Verification items for the finished model (mm, model axes). A direction names the side the tool comes from. Round coordinates to 2 decimals unless told otherwise and drop trailing zeros. Order: outer loops, then holes, each group sorted by start corner. A loop starts at its lowest first (then second) coordinate and runs counter-clockwise, first axis right, second up. Notation, with made-up numbers: M -23.5,53.5 L 32.5,53.5 A15 cw 32.5,62.5 Z; hole C -5,1.5 d11. An arc over 180 degrees is marked long. One line per item, written item: value. Start each with the question number.
from build123d import *

# Parameters (mm, degrees)
F0_R     = 9
F1_DEPTH = 15.3
F2_SIZE  = 1
F3_SIZE2 = 1.5
F3_SIZE  = 1
F4_R     = 3.5
F5_DEPTH = 2
F6_R     = 2.4
F7_DEPTH = 12.5
F8_R     = 1
F9_DEPTH = 1.5


with BuildPart() as f1:
    # F0 (on Top) → F1 (new body)
    with BuildSketch(Plane.XY):
        Circle(F0_R)
    extrude(amount=F1_DEPTH)

    # F2
    f2_edges = [f1.edges().sort_by_distance(p)[0] for p in [
        (-9, 0, 0),
    ]]
    chamfer(f2_edges, length=F2_SIZE)

    # F3
    f3_edges = [f1.edges().sort_by_distance(p)[0] for p in [
        (-9, 0, 15.3),
    ]]
    f3_side = f1.faces().sort_by_distance((0, 0, 15.3))[0]
    chamfer(f3_edges, length=F3_SIZE, length2=F3_SIZE2, reference=f3_side)

    # F4 (on face) → F5 (join)
    with BuildSketch(Plane.XY.offset(15.3)):
        Circle(F4_R)
    extrude(amount=F5_DEPTH)

    # F6 (on face) → F7 (join)
    with BuildSketch(Plane.XY.offset(17.3)):
        Circle(F6_R)
    extrude(amount=F7_DEPTH)

    # F8 (on face) → F9 (join)
    with BuildSketch(Plane(origin=(0, 0, 0), x_dir=(1, 0, 0), z_dir=(0, 0, -1))):
        Circle(F8_R)
    extrude(amount=F9_DEPTH)


solid = f1.part
1. Section check D-D (z = 21.5). Record the cut outline in (x, y), and give its area (3 significant figures).
2. Section check A-A (y = 0). Record the cut outline in (x, z).
3. Depth check by flat-ended pin: pin 1 (6 mm diameter, centred on y = -5.5, z = 21, fed in from +X); pin 2 (4 mm diameter, centred on x = -5, y = -7, fed in from +Z); pin 3 (5 mm diameter, centred on x = 6, y = -2.5, fed in from -Z); pin 4 (1.5 mm diameter, centred on y = 4, z = 15, fed in from +X). Enter the tip coordinate at first touch or a pass-through.
4. Tool access check on faces 1 (the face through (0, 1, -1)), 2 (the face through (1.29, 2.024, 23.462)), 3 (the face through (-1.172, 8.923, 7.31)). Record the directions out of +Z, -Z, +X, -X, +Y, -Y that give a thin tool (end or side, any length) a straight path to the whole face; none if there is none.
5. Scan lines: line 1 along Z through (x, y) = (-7.5, 0.25); line 2 along Z through (x, y) = (-1, 1.75); line 3 along Y through (x, z) = (-3.25, 2). Record each from-to range of solid material in increasing order.
6. Section check C-C (z = 2). Record the cut outline in (x, y), and give its area (3 significant figures).
Geometry check:
1. outline: C 0,0 d4.8
1. area: 18.1 mm²
2. outline: M -9,1 L -8,0 L -1,0 L -1,-1.5 L 1,-1.5 L 1,0 L 8,0 L 9,1 L 9,13.8 L 8,15.3 L 3.5,15.3 L 3.5,17.3 L 2.4,17.3 L 2.4,29.8 L -2.4,29.8 L -2.4,17.3 L -3.5,17.3 L -3.5,15.3 L -8,15.3 L -9,13.8 Z
3. pin 1: passes through
3. pin 2: stops at z = 15.3
3. pin 3: stops at z = 0
3. pin 4: stops at x = 7.84
4. face 1: -Z
4. face 2: +Z
4. face 3: +Z, -Z
5. line 1: z = 0 to 15.3
5. line 2: z = 0 to 29.8
5. line 3: y = -8.39 to 8.39
6. outline: C 0,0 d18
6. area: 254 mm²
